```python
from build123d import *

# Parameters (mm, degrees)
ESTRUSIONE_ESTRUSIONE3_DEPTH = 37
ESTRUSIONE_ESTRUSIONE6_DEPTH = 3
SCHIZZO5_R                   = 2.1
ESTRUSIONE_ESTRUSIONE5_DEPTH = 4
SCHIZZO7_W                   = 6
SCHIZZO7_H                   = 6
TAGLIO_ESTRUSIONE1_DEPTH     = 3


with BuildPart() as part:
    # Schizzo1 → Estrusione-Estrusione3 (new body)
    with BuildSketch(Plane(origin=(0, 0, 0), x_dir=(1, 0, 0), z_dir=(0, 1, 0))):
        Polygon((-18.75, 22.75), (18.75, 22.75), (22.75, 18.75), (22.75, -18.75), (18.75, -22.75), (-18.75, -22.75), (-22.75, -18.75), (-22.75, 18.75), align=None)
        with BuildLine():
            Line((-16.75, 19.75), (16.75, 19.75))
            ThreePointArc((16.75, 19.75), (18.871320344, 18.871320344), (19.75, 16.75))
            Line((19.75, 16.75), (19.75, -16.75))
            ThreePointArc((19.75, -16.75), (18.871320344, -18.871320344), (16.75, -19.75))
            Line((16.75, -19.75), (-16.75, -19.75))
            ThreePointArc((-16.75, -19.75), (-18.871320344, -18.871320344), (-19.75, -16.75))
            Line((-19.75, -16.75), (-19.75, 16.75))
            ThreePointArc((-19.75, 16.75), (-18.871320344, 18.871320344), (-16.75, 19.75))
        make_face(mode=Mode.SUBTRACT)
    extrude(amount=ESTRUSIONE_ESTRUSIONE3_DEPTH)

    # Schizzo6 → Estrusione-Estrusione6 (add)
    with BuildSketch(Plane(origin=(0, 0, 0), x_dir=(1, 0, 0), z_dir=(0, 1, 0))):
        Polygon((-18.75, 22.75), (-22.75, 18.75), (-22.75, -18.75), (-18.75, -22.75), (18.75, -22.75), (22.75, -18.75), (22.75, 18.75), (18.75, 22.75), align=None)
    extrude(amount=ESTRUSIONE_ESTRUSIONE6_DEPTH)

    # Schizzo5 → Estrusione-Estrusione5 (add)
    # profile 1 of 4: a face of its own
    with BuildSketch(Plane(origin=(0, 0, 0), x_dir=(1, 0, 0), z_dir=(0, 1, 0))):
        with BuildLine():
            Line((-22.75, 18.75), (-18.75, 22.75))
            ThreePointArc((-18.75, 22.75), (-20.785786438, 24.048885271), (-21.306854249, 26.406854249))
            ThreePointArc((-21.306854249, 26.406854249), (-30.013098834, 30.013098834), (-26.406854249, 21.306854249))
            ThreePointArc((-26.406854249, 21.306854249), (-24.048885271, 20.785786438), (-22.75, 18.75))
        make_face()
        with Locations(Location((-26.406854249, 26.406854249, 0), (0, 0, 270))):
            Circle(SCHIZZO5_R, mode=Mode.SUBTRACT)
    # profile 2 of 4: a face of its own
    with BuildSketch(Plane(origin=(0, 0, 0), x_dir=(1, 0, 0), z_dir=(0, 1, 0))):
        with BuildLine():
            Line((18.75, 22.75), (22.75, 18.75))
            ThreePointArc((22.75, 18.75), (24.048885271, 20.785786438), (26.406854249, 21.306854249))
            ThreePointArc((26.406854249, 21.306854249), (30.013098834, 30.013098834), (21.306854249, 26.406854249))
            ThreePointArc((21.306854249, 26.406854249), (20.785786438, 24.048885271), (18.75, 22.75))
        make_face()
        with Locations(Location((26.406854249, 26.406854249, 0), (0, 0, 270))):
            Circle(SCHIZZO5_R, mode=Mode.SUBTRACT)
    # profile 3 of 4: a face of its own
    with BuildSketch(Plane(origin=(0, 0, 0), x_dir=(1, 0, 0), z_dir=(0, 1, 0))):
        with BuildLine():
            Line((22.75, -18.75), (18.75, -22.75))
            ThreePointArc((18.75, -22.75), (20.785786438, -24.048885271), (21.306854249, -26.406854249))
            ThreePointArc((21.306854249, -26.406854249), (30.013098834, -30.013098834), (26.406854249, -21.306854249))
            ThreePointArc((26.406854249, -21.306854249), (24.048885271, -20.785786438), (22.75, -18.75))
        make_face()
        with Locations(Location((26.406854249, -26.406854249, 0), (0, 0, 270))):
            Circle(SCHIZZO5_R, mode=Mode.SUBTRACT)
    # profile 4 of 4: a face of its own
    with BuildSketch(Plane(origin=(0, 0, 0), x_dir=(1, 0, 0), z_dir=(0, 1, 0))):
        with BuildLine():
            Line((-18.75, -22.75), (-22.75, -18.75))
            ThreePointArc((-22.75, -18.75), (-24.048885271, -20.785786438), (-26.406854249, -21.306854249))
            ThreePointArc((-26.406854249, -21.306854249), (-30.013098834, -30.013098834), (-21.306854249, -26.406854249))
            ThreePointArc((-21.306854249, -26.406854249), (-20.785786438, -24.048885271), (-18.75, -22.75))
        make_face()
        with Locations(Location((-26.406854249, -26.406854249, 0), (0, 0, 270))):
            Circle(SCHIZZO5_R, mode=Mode.SUBTRACT)
    extrude(amount=ESTRUSIONE_ESTRUSIONE5_DEPTH)

    # Schizzo7 → Taglio-Estrusione1 (cut)
    with BuildSketch(Plane.XY.offset(22.75)):
        with Locations((0, 10)):
            Rectangle(SCHIZZO7_W, SCHIZZO7_H)
    extrude(amount=-TAGLIO_ESTRUSIONE1_DEPTH, mode=Mode.SUBTRACT)


solid = part.part
```
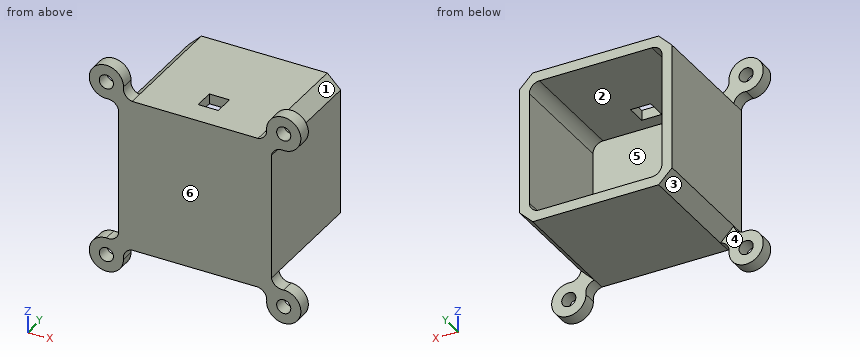
CAD build for the part. Positions are in the model's coordinates, mm. Face numbers are marked on the shaded views. A direction names the side the tool comes from. Coordinates: 2 decimals unless noted, no trailing zeros. Write each loop counter-clockwise with the first axis right and the second up, starting at its lowest first coordinate (ties: lowest second). Pieces come first, ordered by that corner, then holes.
(1) Drill centre lines: probe 1 along Z at (x, y) = (4, 13); probe 2 along Z at (x, y) = (17, 17). Where is each one in solid material? Low to high.
(2) Two-plate mould, pull along X, no slides. Class the marked faces 1, 2 and 3: +X half, -X half, draft (parallel to the pull), parting line (faces both ways), or undercut.
(3) Cut at B-B, the plane x = 15. List the corners of the cut face in (y, z).
(4) 3-axis set-ups, long thin cutter, end or side, ignore diameter. For the marked faces 4, 5 and 6: which of +Z, -Z, +X, -X, +Y, -Y reach the whole face in a straight line?
(5) Flat gauge pins, fed straight in: pin 1 (2.5 mm diameter, centred on y = 11, z = 21.5, fed in from +X); pin 2 (10 mm diameter, centred on y = 9.5, z = -21, fed in from +X); pin 3 (10 mm diameter, centred on x = 4, y = 30, fed in from -Z); pin 4 (14 mm diameter, centred on x = 26, z = -25, fed in from +Y). Where does each tip first touch, or does it go through?
(6) Cut at D-D, the plane y = 9. List the corners of the cut face in (x, z), and give its area (3 significant figures).
(7) Cut at A-A, the plane y = 15.5. List the corners of the cut face in (x, z).
(8) Cut at C-C, the plane z = -2. List the corners of the cut face in (x, y).
Geometry says:
1. probe 1: z = -22.75 to -19.75, 19.75 to 22.75
1. probe 2: z = -22.75 to -19.74, 19.74 to 22.75
2. face 1: +X half
2. face 2: undercut
2. face 3: -X half
3. outline: (0, -22.75) - (37, -22.75) - (37, -19.75) - (3, -19.75) - (3, 19.75) - (37, 19.75) - (37, 22.75) - (0, 22.75) - close
4. face 4: -Z, -X, +Y
4. face 5: +Y
4. face 6: +Z, -Z, +X, -X, -Y
5. pin 1: stops at x = 21.25
5. pin 2: stops at x = 22.75
5. pin 3: stops at z = -22.75
5. pin 4: stops at y = 37
6. outline: (-22.75, -18.75) - (-18.75, -22.75) - (18.75, -22.75) - (22.75, -18.75) - (22.75, 18.75) - (18.75, 22.75) - (3, 22.75) - (3, 19.75) - (16.75, 19.75) arc R3 cw to (19.75, 16.75) - (19.75, -16.75) arc R3 cw to (16.75, -19.75) - (-16.75, -19.75) arc R3 cw to (-19.75, -16.75) - (-19.75, 16.75) arc R3 cw to (-16.75, 19.75) - (-3, 19.75) - (-3, 22.75) - (-18.75, 22.75) - (-22.75, 18.75) - close
6. area: 468 mm2
7. outline: (-22.75, -18.75) - (-18.75, -22.75) - (18.75, -22.75) - (22.75, -18.75) - (22.75, 18.75) - (18.75, 22.75) - (-18.75, 22.75) - (-22.75, 18.75) - close; hole (-19.75, -16.75) arc R3 ccw to (-16.75, -19.75) - (16.75, -19.75) arc R3 ccw to (19.75, -16.75) - (19.75, 16.75) arc R3 ccw to (16.75, 19.75) - (-16.75, 19.75) arc R3 ccw to (-19.75, 16.75) - close
8. outline: (-22.75, 0) - (22.75, 0) - (22.75, 37) - (19.75, 37) - (19.75, 3) - (-19.75, 3) - (-19.75, 37) - (-22.75, 37) - close
